Design review of the part built by this model. Coordinates are the model's own, in mm. Face numbers are marked on the shaded views. A direction names the side the tool comes from. Coordinates: 2 decimals unless noted, no trailing zeros. Write each loop counter-clockwise with the first axis right and the second up, starting at its lowest first coordinate (ties: lowest second). Pieces come first, ordered by that corner, then holes.
Q1. Take a section at C-C (x = 0). Give the boundary of the cut face in (y, z).
Q2. For probe 1 along Z at (x, y) = (0.5, -1.5); probe 2 along Z at (x, y) = (2.5, 1.5); probe 3 along Y at (x, z) = (2, 9.5), list the stretches that pass through material, from the lowest coordinate up.
Q3. Insertion check: pin 1 (1.5 mm diameter, centred on x = 3, y = -3.5, fed in from +Z); pin 2 (3 mm diameter, centred on x = -3, z = 49.5, fed in from +Y); pin 3 (1.5 mm diameter, centred on y = 0.5, z = 19, fed in from +X). Each pin has a flat end and moves straight along its axis. Give the tip position at first contact, or say it passes through.
Q4. Machinability: for the marked faces 1 and 2, which of the approach directions +Z, -Z, +X, -X, +Y, -Y give a long, thin tool a straight path to every point of the face, cutting with its end or side? Answer none if there is none.
Q5. Take a section at D-D (z = 14). Give the boundary of the cut face in (x, y).
Q6. Take a section at B-B (y = 0). Give the boundary of the cut face in (x, z).
Q7. Take a section at A-A (z = 3). Give the boundary of the cut face in (x, y), and give its area (3 significant figures).
```python
from build123d import *

# Parameters (mm, degrees)
F0_R     = 6
F1_DEPTH = 15
F2_R     = 4
F3_DEPTH = 20
F4_R     = 2
F5_DEPTH = 23
F6_R     = 0.5
F8_DEPTH = 10


with BuildPart() as f1:
    # F0 (on Top) → F1 (new body)
    with BuildSketch(Plane.XY):
        Circle(F0_R)
    extrude(amount=F1_DEPTH)

    # F2 (on face) → F3 (join)
    with BuildSketch(Plane.XY.offset(15)):
        Circle(F2_R)
    extrude(amount=F3_DEPTH)

    # F4 (on face) → F5 (join)
    with BuildSketch(Plane.XY.offset(35)):
        Circle(F4_R)
    extrude(amount=F5_DEPTH)

    # F6
    f6_edges = [f1.edges().sort_by_distance(p)[0] for p in [
        (-4, 0, 35),
        (-6, 0, 15),
        (-2, 0, 58),
    ]]
    fillet(f6_edges, radius=F6_R)

    # F7 (on face) → F8 (cut)
    with BuildSketch(Plane(origin=(0, 0, 0), x_dir=(1, 0, 0), z_dir=(0, 0, -1))):
        with BuildLine():
            ThreePointArc((-1.658312, 2.5), (-3, 0), (-1.658312, -2.5))
            Line((-1.658312, -2.5), (1.658312, -2.5))
            ThreePointArc((1.658312, -2.5), (3, 0), (1.658312, 2.5))
            Line((1.658312, 2.5), (-1.658312, 2.5))
        make_face()
    extrude(amount=-F8_DEPTH, mode=Mode.SUBTRACT)


solid = f1.part
```
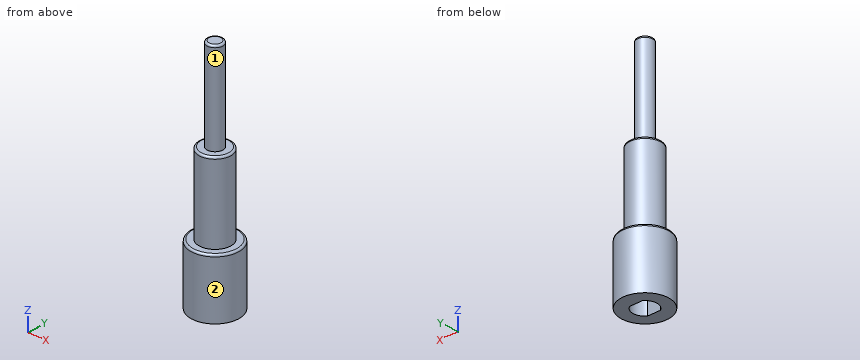
Response:
1. outline: (-6, 0) - (-2.5, 0) - (-2.5, 10) - (2.5, 10) - (2.5, 0) - (6, 0) - (6, 14.5) arc R0.5 ccw to (5.5, 15) - (4, 15) - (4, 34.5) arc R0.5 ccw to (3.5, 35) - (2, 35) - (2, 57.5) arc R0.5 ccw to (1.5, 58) - (-1.5, 58) arc R0.5 ccw to (-2, 57.5) - (-2, 35) - (-3.5, 35) arc R0.5 ccw to (-4, 34.5) - (-4, 15) - (-5.5, 15) arc R0.5 ccw to (-6, 14.5) - close
2. probe 1: z = 10 to 57.99
2. probe 2: z = 10 to 35
2. probe 3: y = -5.66 to -2.24, 2.24 to 5.66
3. pin 1: stops at z = 34.85
3. pin 2: stops at y = 1.32
3. pin 3: stops at x = 4
4. face 1: +Z
4. face 2: +Z, -Z
5. outline: circle Ø12 at (0, 0)
6. outline: (-6, 0) - (-3, 0) - (-3, 10) - (3, 10) - (3, 0) - (6, 0) - (6, 14.5) arc R0.5 ccw to (5.5, 15) - (4, 15) - (4, 34.5) arc R0.5 ccw to (3.5, 35) - (2, 35) - (2, 57.5) arc R0.5 ccw to (1.5, 58) - (-1.5, 58) arc R0.5 ccw to (-2, 57.5) - (-2, 35) - (-3.5, 35) arc R0.5 ccw to (-4, 34.5) - (-4, 15) - (-5.5, 15) arc R0.5 ccw to (-6, 14.5) - close
7. outline: circle Ø12 at (0, 0); hole (-1.66, -2.5) - (1.66, -2.5) arc R3 ccw to (1.66, 2.5) - (-1.66, 2.5) arc R3 ccw to start
7. area: 87.1 mm2
